Read the model definition and answer for the solid it produces. Units are mm, in the model's axes. Face numbers are marked on the shaded views. A direction names the side the tool comes from. Coordinates: 2 decimals unless noted, no trailing zeros. Order: outer loops, then holes, each group sorted by start corner. A loop starts at its lowest first (then second) coordinate and runs counter-clockwise, first axis right, second up. Notation, with made-up numbers: (39, -9.75) -> (83, -9.75) arc R21 ccw to (83, 18.25) -> close; hole circle Ø11 at (15, 75). An arc over 180 degrees is marked (long way). Return JSON: item names as keys, results as strings. Group by question number.
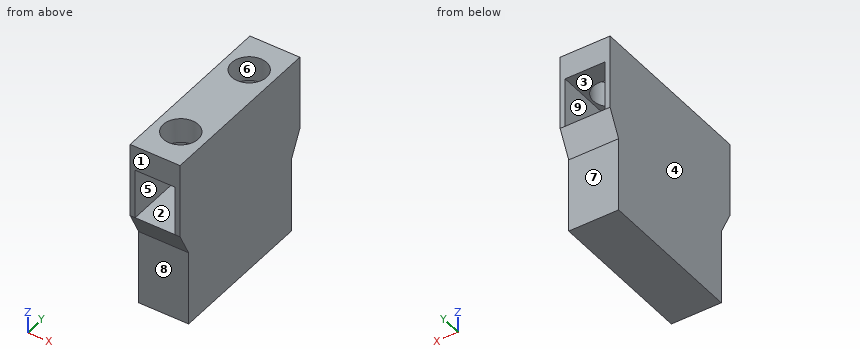
```python
from build123d import *

# Parameters (mm, degrees)
SKETCH1_W           = 15
SKETCH1_H           = 30
BOSS_EXTRUDE1_DEPTH = 10
SKETCH2_R           = 3.5
CUT_EXTRUDE1_DEPTH  = 15
SKETCH3_W           = 8
SKETCH3_H           = 10
CUT_EXTRUDE2_DEPTH  = 35
SKETCH4_W           = 10
SKETCH4_H           = 5
BOSS_EXTRUDE2_DEPTH = 35


with BuildPart() as part:
    # Sketch1 → Boss-Extrude1 (new body)
    with BuildSketch(Plane(origin=(0, 0, 0), x_dir=(0, 0, -1), z_dir=(1, 0, 0))):
        with Locations((27.5, 17.5)):
            Rectangle(SKETCH1_W, SKETCH1_H)
        Polygon((20, 2.5), (20, 32.5), (15, 35), (0, 35), (0, 0), (15, 0), align=None)
    extrude(amount=BOSS_EXTRUDE1_DEPTH)

    # Sketch2 → Cut-Extrude1 (cut)
    with BuildSketch(Plane.XY):
        with Locations((5, 27.5)):
            Circle(SKETCH2_R)
        with Locations((5, 7.5)):
            Circle(SKETCH2_R)
    extrude(amount=-CUT_EXTRUDE1_DEPTH, mode=Mode.SUBTRACT)

    # Sketch3 → Cut-Extrude2 (cut)
    with BuildSketch(Plane(origin=(0, 35, 0), x_dir=(1, 0, 0), z_dir=(0, 1, 0))):
        with Locations((5, 10)):
            Rectangle(SKETCH3_W, SKETCH3_H)
    extrude(amount=-CUT_EXTRUDE2_DEPTH, mode=Mode.SUBTRACT)

    # Sketch4 → Boss-Extrude2 (add)
    with BuildSketch(Plane.XY):
        with Locations((5, 17.5)):
            Rectangle(SKETCH4_W, SKETCH4_H)
    extrude(amount=-BOSS_EXTRUDE2_DEPTH)


solid = part.part
```
1. Find section D-D on x = 2.5. Determine the outline of the cut face in (y, z), and give its area (3 significant figures).
2. Which of the six approach directions +Z, -Z, +X, -X, +Y, -Y give full straight-line access (tool end or side, diameter ignored) to the marked faces 5, 6, 7, 8 and 9?
3. Find section C-C on z = -7. Determine the outline of the cut face in (x, y), and give its area (3 significant figures).
4. Straight lines are drawn through the part: L1, parallel to Y at x = 5, z = -3; L2, parallel to Z at x = 7, y = 23; L3, parallel to Z at x = 2.5, y = 6. For each, find the intervals that lie inside material, in ascending order.
5. Find section A-A on x = 5. Determine the outline of the cut face in (y, z), and give its area (4 significant figures).
6. For a pull along X with two mould halves and no side action, classify the marked faces 1, 2, 3 and 4 as released by +X, released by -X, zero draft, split by the parting line, or undercut.
7. Find section B-B on y = 27.5. Determine the outline of the cut face in (x, z).
8. Given pin 1 (4 mm diameter, centred on x = 4, z = -10.5, fed in from +Y); pin 2 (3 mm diameter, centred on x = 6.5, y = 8.5, fed in from +Z); pin 3 (2.5 mm diameter, centred on x = 7, z = -9, fed in from -Y), each flat-ended and moving along its own axis, determine where each tip first touches the part or whether it passes through.
Result:
{
 "1": {"outline": "(0, -15) -> (2.5, -20) -> (2.5, -35) -> (32.5, -35) -> (32.5, -20) -> (35, -15) -> (20, -15) -> (20, -5) -> (25.05, -5) -> (25.05, 0) -> (9.95, 0) -> (9.95, -5) -> (15, -5) -> (15, -15) -> close; (0, -5) -> (5.05, -5) -> (5.05, 0) -> (0, 0) -> close; (29.95, -5) -> (35, -5) -> (35, 0) -> (29.95, 0) -> close", "area": "789 mm^2"},
 "2": {"face 5": "-Y", "face 6": "+Z", "face 7": "-Z, +X, -X, +Y", "face 8": "-Z, +X, -X, -Y", "face 9": "+Y"},
 "3": {"outline": "(0, 0) -> (1, 0) -> (1, 15) -> (9, 15) -> (9, 0) -> (10, 0) -> (10, 35) -> (9, 35) -> (9, 20) -> (1, 20) -> (1, 35) -> (0, 35) -> close", "area": "110 mm^2"},
 "4": {"L1": "0 to 4, 11 to 24, 31 to 35", "L2": "-35 to -15, -5 to 0", "L3": "-35 to -15"},
 "5": {"outline": "(0, -15) -> (2.5, -20) -> (2.5, -35) -> (32.5, -35) -> (32.5, -20) -> (35, -15) -> (20, -15) -> (20, -5) -> (24, -5) -> (24, 0) -> (11, 0) -> (11, -5) -> (15, -5) -> (15, -15) -> close; (0, -5) -> (4, -5) -> (4, 0) -> (0, 0) -> close; (31, -5) -> (35, -5) -> (35, 0) -> (31, 0) -> close", "area": "767.5 mm^2"},
 "6": {"face 1": "zero draft", "face 2": "undercut", "face 3": "undercut", "face 4": "released by -X"},
 "7": {"outline": "(0, -35) -> (10, -35) -> (10, 0) -> (8.5, 0) -> (8.5, -5) -> (9, -5) -> (9, -15) -> (1, -15) -> (1, -5) -> (1.5, -5) -> (1.5, 0) -> (0, 0) -> close"},
 "8": {"pin 1": "y = 20", "pin 2": "z = -15", "pin 3": "y = 15"}
}
